```python
from build123d import *

# Parameters (mm, degrees)
BASE_FLANGE1_DEPTH        = 132
HEM2_START                = -107
HEM2_DEPTH                = 96.2
SKETCH31_R                = 12.7
CUT_EXTRUDE1_DEPTH        = 208.181817916
EDGE_FLANGE1_DEPTH        = 96.2
EDGE_FLANGE1_BEND_DEPTH   = 213.4
EDGE_FLANGE1_BEND_2_DEPTH = 96.2
CHAMFER1_SIZE             = 7
SKETCH41_W                = 21.5
SKETCH41_H                = 27.5
CUT_EXTRUDE2_DEPTH        = 208.181817916
LPATTERN1_COUNT           = 3
LPATTERN1_PITCH           = 33.5
SKETCH44_W                = 235
SKETCH44_H                = 10
CUT_EXTRUDE3_DEPTH        = 0.1
EDGE_FLANGE2_DEPTH        = 123.325
EDGE_FLANGE2_START        = 122.925
EDGE_FLANGE2_2_DEPTH      = 0.4
EDGE_FLANGE2_3_DEPTH      = 122.925
EDGE_FLANGE4_START        = -106.9
EDGE_FLANGE4_DEPTH        = 96.1
EDGE_FLANGE4_2_DEPTH      = 96.1
CHAMFER2_SIZE             = 6
SKETCH80_W                = 213.4
SKETCH80_H                = 1
BOSS_EXTRUDE1_DEPTH       = 7
FILLET1_R                 = 1
SKETCH92_W                = 37
SKETCH92_H                = 27.5
CUT_EXTRUDE4_DEPTH        = 208.181817916


# Read off the part's stored shape, not the designer's step: Hem2, Edge-Flange2, Edge-Flange4
# Sheet-metal steps are written as plain solids
with BuildPart() as part:
    # Sketch1 → Base-Flange1 (new body)
    with BuildSketch(Plane(origin=(0, 0, 0), x_dir=(1, 0, 0), z_dir=(0, 1, 0))):
        with BuildLine():
            Line((117.5, 107), (117.5, 10.8))
            ThreePointArc((117.5, 10.8), (114.336753237, 3.163246763), (106.7, 0))
            Line((106.7, 0), (0, 0))
            Line((0, 0), (-106.7, 0))
            ThreePointArc((-106.7, 0), (-114.336753237, 3.163246763), (-117.5, 10.8))
            Line((-117.5, 10.8), (-117.5, 107))
            Line((-117.5, 107), (-116.7, 107))
            Line((-116.7, 107), (-116.7, 10.8))
            ThreePointArc((-116.7, 10.8), (-113.771067812, 3.728932188), (-106.7, 0.8))
            Line((-106.7, 0.8), (0, 0.8))
            Line((0, 0.8), (106.7, 0.8))
            ThreePointArc((106.7, 0.8), (113.771067812, 3.728932188), (116.7, 10.8))
            Line((116.7, 10.8), (116.7, 107))
            Line((116.7, 107), (117.5, 107))
        make_face()
    extrude(amount=BASE_FLANGE1_DEPTH)

    # Hem2 outline → Hem2 (add)
    with BuildSketch(Plane.XY.offset(HEM2_START)):
        with BuildLine():
            Line((-116.45, 123.925), (-115.65, 123.925))
            Line((-115.65, 123.925), (-115.65, 132))
            ThreePointArc((-115.65, 132), (-116.575, 132.925), (-117.5, 132))
            Line((-117.5, 132), (-116.7, 132))
            ThreePointArc((-116.7, 132), (-116.575, 132.125), (-116.45, 132))
            Line((-116.45, 132), (-116.45, 123.925))
        make_face()
        with BuildLine():
            Line((115.65, 123.925), (116.45, 123.925))
            Line((116.45, 123.925), (116.45, 132))
            ThreePointArc((116.45, 132), (116.575, 132.125), (116.7, 132))
            Line((116.7, 132), (117.5, 132))
            ThreePointArc((117.5, 132), (116.575, 132.925), (115.65, 132))
            Line((115.65, 132), (115.65, 123.925))
        make_face()
    extrude(amount=HEM2_DEPTH)

    # Sweep1: sweep along a path in Sketch30
    with BuildLine(Plane(origin=(0, 132, 0), x_dir=(1, 0, 0), z_dir=(0, 1, 0))) as sweep1_path:
        ThreePointArc((-116.7, 10.8), (-113.771067812, 3.728932188), (-106.7, 0.8))
        Line((-106.7, 0.8), (106.7, 0.8))
        ThreePointArc((106.7, 0.8), (113.771067812, 3.728932188), (116.7, 10.8))
    # Sketch29 → Sweep1 (sweep)
    with BuildSketch(Plane.XY.offset(-10.8)):
        with BuildLine():
            Line((-117.5, 132), (-116.7, 132))
            ThreePointArc((-116.7, 132), (-116.575, 132.125), (-116.45, 132))
            Line((-116.45, 132), (-116.45, 123.925))
            Line((-116.45, 123.925), (-115.65, 123.925))
            Line((-115.65, 123.925), (-115.65, 132))
            ThreePointArc((-115.65, 132), (-116.575, 132.925), (-117.5, 132))
        make_face()
    sweep(path=sweep1_path.line)

    # Sketch31 → Cut-Extrude1 (cut, through all)
    with BuildSketch(Plane.XY):
        with Locations((87, 35.2)):
            Circle(SKETCH31_R)
    extrude(amount=-CUT_EXTRUDE1_DEPTH, mode=Mode.SUBTRACT)

    # Edge-Flange1 section (across the edge) → Edge-Flange1 (add)
    with BuildSketch(Plane(origin=(-116.7, -1, -10.8), x_dir=(0, 1, 0), z_dir=(0, 0, -1))):
        with BuildLine():
            Line((-0.8, 1), (-0.8, 7.5))
            Line((-0.8, 7.5), (0, 7.5))
            Line((0, 7.5), (0, 1))
            ThreePointArc((0, 1), (0.292893219, 0.292893219), (1, 0))
            Line((1, 0), (1, -0.8))
            ThreePointArc((1, -0.8), (-0.272792206, -0.272792206), (-0.8, 1))
        make_face()
    extrude(amount=EDGE_FLANGE1_DEPTH)

    # Edge-Flange1 section 2 (across the edge) → Edge-Flange1 bend (add)
    with BuildSketch(Plane(origin=(106.7, -1, -0.8), x_dir=(0, 1, 0), z_dir=(-1, 0, 0))):
        with BuildLine():
            Line((-0.8, 1), (-0.8, 7.5))
            Line((-0.8, 7.5), (0, 7.5))
            Line((0, 7.5), (0, 1))
            ThreePointArc((0, 1), (0.292893219, 0.292893219), (1, 0))
            Line((1, 0), (1, -0.8))
            ThreePointArc((1, -0.8), (-0.272792206, -0.272792206), (-0.8, 1))
        make_face()
    extrude(amount=EDGE_FLANGE1_BEND_DEPTH)

    # Edge-Flange1 section 3 (across the edge) → Edge-Flange1 bend 2 (add)
    with BuildSketch(Plane(origin=(116.7, -1, -107), x_dir=(0, 1, 0), z_dir=(0, 0, 1))):
        with BuildLine():
            Line((-0.8, 1), (-0.8, 7.5))
            Line((-0.8, 7.5), (0, 7.5))
            Line((0, 7.5), (0, 1))
            ThreePointArc((0, 1), (0.292893219, 0.292893219), (1, 0))
            Line((1, 0), (1, -0.8))
            ThreePointArc((1, -0.8), (-0.272792206, -0.272792206), (-0.8, 1))
        make_face()
    extrude(amount=EDGE_FLANGE1_BEND_2_DEPTH)

    # Chamfer1
    chamfer1_edges = [part.edges().sort_by_distance(p)[0] for p in [
        (106.7, -1.4, -8.3),
        (109.2, -1.4, -10.8),
        (-106.7, -1.4, -8.3),
        (-109.2, -1.4, -10.8),
    ]]
    chamfer(chamfer1_edges, length=CHAMFER1_SIZE)

    # Sketch41 → Cut-Extrude2 (cut, through all)
    with BuildSketch(Plane.XY):
        with Locations((-73.45, 102.6)):
            Rectangle(SKETCH41_W, SKETCH41_H)
    cut_extrude2 = extrude(amount=-CUT_EXTRUDE2_DEPTH, mode=Mode.SUBTRACT)

    # LPattern1: Cut-Extrude2 ×3
    with Locations(*[(0, -i * LPATTERN1_PITCH, 0) for i in range(1, LPATTERN1_COUNT)]):
        add(cut_extrude2, mode=Mode.SUBTRACT)

    # Sketch44 → Cut-Extrude3 (cut)
    with BuildSketch(Plane(origin=(0, 0, -107), x_dir=(-1, 0, 0), z_dir=(0, 0, -1))):
        with Locations((0, 127.925)):
            Rectangle(SKETCH44_W, SKETCH44_H)
    extrude(amount=-CUT_EXTRUDE3_DEPTH, mode=Mode.SUBTRACT)

    # Edge-Flange2 outline → Edge-Flange2 (cut)
    with BuildSketch(Plane(origin=(0, 0, 0), x_dir=(1, 0, 0), z_dir=(0, 1, 0))):
        with BuildLine():
            ThreePointArc((116.7, 105.662741699), (117.29411255, 104.6), (117.5, 103.4))
            Line((117.5, 103.4), (117.5, 107))
            Line((117.5, 107), (116.7, 107))
            Line((116.7, 107), (116.7, 105.662741699))
        make_face()
        with BuildLine():
            ThreePointArc((-117.5, 103.4), (-117.29411255, 104.6), (-116.7, 105.662741699))
            Line((-116.7, 105.662741699), (-116.7, 107))
            Line((-116.7, 107), (-117.5, 107))
            Line((-117.5, 107), (-117.5, 103.4))
        make_face()
    extrude(amount=EDGE_FLANGE2_DEPTH, mode=Mode.SUBTRACT)

    # Edge-Flange2 2 outline → Edge-Flange2 2 (cut)
    with BuildSketch(Plane(origin=(0, 0, 0), x_dir=(1, 0, 0), z_dir=(0, 1, 0)).offset(EDGE_FLANGE2_START)):
        with BuildLine():
            ThreePointArc((117.5, 103.4), (117.29411255, 104.6), (116.7, 105.662741699))
            Line((116.7, 105.662741699), (116.7, 103))
            Line((116.7, 103), (117.5, 103))
            Line((117.5, 103), (117.5, 103.4))
        make_face()
        with BuildLine():
            Line((-116.7, 103), (-116.7, 105.662741699))
            ThreePointArc((-116.7, 105.662741699), (-117.29411255, 104.6), (-117.5, 103.4))
            Line((-117.5, 103.4), (-117.5, 103))
            Line((-117.5, 103), (-116.7, 103))
        make_face()
    extrude(amount=EDGE_FLANGE2_2_DEPTH, mode=Mode.SUBTRACT)

    # Edge-Flange2 3 outline → Edge-Flange2 3 (add)
    with BuildSketch(Plane(origin=(0, 0, 0), x_dir=(1, 0, 0), z_dir=(0, 1, 0))):
        with BuildLine():
            Line((113.9, 107), (101.7, 107))
            Line((101.7, 107), (101.7, 106.2))
            Line((101.7, 106.2), (113.9, 106.2))
            ThreePointArc((113.9, 106.2), (115.879898987, 105.379898987), (116.7, 103.4))
            Line((116.7, 103.4), (116.7, 105.662741699))
            ThreePointArc((116.7, 105.662741699), (115.451471863, 106.648528137), (113.9, 107))
        make_face()
        with BuildLine():
            Line((-101.7, 107), (-113.9, 107))
            ThreePointArc((-113.9, 107), (-115.451471863, 106.648528137), (-116.7, 105.662741699))
            Line((-116.7, 105.662741699), (-116.7, 103.4))
            ThreePointArc((-116.7, 103.4), (-115.879898987, 105.379898987), (-113.9, 106.2))
            Line((-113.9, 106.2), (-101.7, 106.2))
            Line((-101.7, 106.2), (-101.7, 107))
        make_face()
    extrude(amount=EDGE_FLANGE2_3_DEPTH)

    # Edge-Flange4 outline → Edge-Flange4 (cut)
    with BuildSketch(Plane.XY.offset(EDGE_FLANGE4_START)):
        with BuildLine():
            ThreePointArc((116.45, 125.725), (116.237450787, 124.876471863), (115.65, 124.228337046))
            Line((115.65, 124.228337046), (115.65, 123.925))
            Line((115.65, 123.925), (116.45, 123.925))
            Line((116.45, 123.925), (116.45, 125.725))
        make_face()
        with BuildLine():
            Line((-115.65, 123.925), (-115.65, 124.228337046))
            ThreePointArc((-115.65, 124.228337046), (-116.237450787, 124.876471863), (-116.45, 125.725))
            Line((-116.45, 125.725), (-116.45, 123.925))
            Line((-116.45, 123.925), (-115.65, 123.925))
        make_face()
    extrude(amount=EDGE_FLANGE4_DEPTH, mode=Mode.SUBTRACT)

    # Edge-Flange4 2 outline → Edge-Flange4 2 (add)
    with BuildSketch(Plane.XY.offset(EDGE_FLANGE4_START)):
        with BuildLine():
            Line((109.45, 123.925), (114.65, 123.925))
            ThreePointArc((114.65, 123.925), (115.172497216, 124.002502784), (115.65, 124.228337046))
            Line((115.65, 124.228337046), (115.65, 125.725))
            ThreePointArc((115.65, 125.725), (115.357106781, 125.017893219), (114.65, 124.725))
            Line((114.65, 124.725), (109.45, 124.725))
            Line((109.45, 124.725), (109.45, 123.925))
        make_face()
        with BuildLine():
            Line((-114.65, 123.925), (-109.45, 123.925))
            Line((-109.45, 123.925), (-109.45, 124.725))
            Line((-109.45, 124.725), (-114.65, 124.725))
            ThreePointArc((-114.65, 124.725), (-115.357106781, 125.017893219), (-115.65, 125.725))
            Line((-115.65, 125.725), (-115.65, 124.228337046))
            ThreePointArc((-115.65, 124.228337046), (-115.172497216, 124.002502784), (-114.65, 123.925))
        make_face()
    extrude(amount=EDGE_FLANGE4_2_DEPTH)

    # Chamfer2
    chamfer2_edges = [part.edges().sort_by_distance(p)[0] for p in [
        (-109.45, 124.325, -10.8),
        (109.45, 124.325, -10.8),
    ]]
    chamfer(chamfer2_edges, length=CHAMFER2_SIZE)

    # Sketch80 → Boss-Extrude1 (add)
    with BuildSketch(Plane(origin=(0, 0, -1.85), x_dir=(-1, 0, 0), z_dir=(0, 0, -1))):
        with Locations((0, 124.425)):
            Rectangle(SKETCH80_W, SKETCH80_H)
    extrude(amount=BOSS_EXTRUDE1_DEPTH)

    # Fillet1
    fillet1_edges = [part.edges().sort_by_distance(p)[0] for p in [
        (0, 124.925, -1.85),
    ]]
    fillet(fillet1_edges, radius=FILLET1_R)

    # Sketch92 → Cut-Extrude4 (cut, through all)
    with BuildSketch(Plane.XY):
        with Locations((-10.7, 102.6)):
            Rectangle(SKETCH92_W, SKETCH92_H)
    extrude(amount=-CUT_EXTRUDE4_DEPTH, mode=Mode.SUBTRACT)


solid = part.part
```
For this review, take the finished solid that the model builds, in its own axes (mm). A direction names the side the tool comes from. Coordinates: 2 decimals unless noted, no trailing zeros. Write each loop counter-clockwise with the first axis right and the second up, starting at its lowest first coordinate (ties: lowest second). Pieces come first, ordered by that corner, then holes. Notation, with made-up numbers: (-3.5, -14.5) - (16.5, -14.5) arc R15 ccw to (16.5, 3.5) - close; hole circle Ø10 at (-28.75, 76). An arc over 180 degrees is marked (long way). Answer in a Markdown table with one row per item. Add a question column.
Q1. We need section D-D, the plane y = 65. State the section outline as (x, z) points, and give its area (3 significant figures).
Q2. We need section A-A, the plane y = 35.2. State the section outline as (x, z) points, and give its area (3 significant figures).
Q3. Tool access review of faces 4 (the flat face through (1, 128, -1.05)), 5 (the cylindrical face through (-113.67, 127.91, -3.98)), 6 (the flat face through (112, 124.725, -60)), 7 (the flat face through (112, -1, -60)): name each direction out of +Z, -Z, +X, -X, +Y, -Y from which nothing blocks a thin tool from reaching the whole face with its end or side.
Q4. For P1, Ø1.6, axis at y = 125, z = -6.5, coming from the -X side; P2, Ø3, axis at x = 112.5, z = -3, coming from the -Y side; P3, Ø2, axis at x = -85, y = 98, coming from the -Z side; P4, Ø23, axis at x = 87, y = 35.2, coming from the -Z side, all flat-tipped, find the tip position at first contact; note any pin that passes through.
Q5. For probe 1 along Y at (x, z) = (88, -6) (3 decimals); probe 2 along X at (y, z) = (12.5, -14); probe 3 along Y at (x, z) = (87, -0.6), list the stretches that pass through material, from the lowest coordinate up.
Q6. Draft analysis for pull direction X (two halves, no side actions). For faces 1 (the flat face through (116, 127, -106.9)), 2 (the flat face through (-103.2, -1.4, -4.8)), 3 (the flat face through (-112.7, -1.4, -14.3)), state which applies: +X half, -X half, draft (parallel to the pull), parting line (faces both ways), or undercut.
Q7. We need section C-C, the plane x = 2. State the section outline as (y, z) points (3 decimals), and give its area (3 significant figures).
Answer list:
| question | item | result |
|---|---|---|
| 1 | outline | (-117.5, -103.4) arc R3.6 ccw to (-113.9, -107) - (-101.7, -107) - (-101.7, -106.2) - (-113.9, -106.2) arc R2.8 cw to (-116.7, -103.4) - (-116.7, -10.8) arc R10 cw to (-106.7, -0.8) - (-84.2, -0.8) - (-84.2, 0) - (-106.7, 0) arc R10.8 ccw to (-117.5, -10.8) - close; (-62.7, -0.8) - (106.7, -0.8) arc R10 cw to (116.7, -10.8) - (116.7, -103.4) arc R2.8 cw to (113.9, -106.2) - (101.7, -106.2) - (101.7, -107) - (113.9, -107) arc R3.6 ccw to (117.5, -103.4) - (117.5, -10.8) arc R10.8 ccw to (106.7, 0) - (-62.7, 0) - close |
| 1 | area | 355 mm2 |
| 2 | outline | (-117.5, -103.4) arc R3.6 ccw to (-113.9, -107) - (-101.7, -107) - (-101.7, -106.2) - (-113.9, -106.2) arc R2.8 cw to (-116.7, -103.4) - (-116.7, -10.8) arc R10 cw to (-106.7, -0.8) - (-84.2, -0.8) - (-84.2, 0) - (-106.7, 0) arc R10.8 ccw to (-117.5, -10.8) - close; (-62.7, -0.8) - (74.3, -0.8) - (74.3, 0) - (-62.7, 0) - close; (99.7, -0.8) - (106.7, -0.8) arc R10 cw to (116.7, -10.8) - (116.7, -103.4) arc R2.8 cw to (113.9, -106.2) - (101.7, -106.2) - (101.7, -107) - (113.9, -107) arc R3.6 ccw to (117.5, -103.4) - (117.5, -10.8) arc R10.8 ccw to (106.7, 0) - (99.7, 0) - close |
| 2 | area | 335 mm2 |
| 3 | face 4 | none |
| 3 | face 5 | -Y |
| 3 | face 6 | -Z, +Y |
| 3 | face 7 | +Z, -Z |
| 4 | P1 | stops at x = -116.92 |
| 4 | P2 | stops at y = 0 |
| 4 | P3 | stops at z = -0.8 |
| 4 | P4 | passes through |
| 5 | probe 1 | y = -1.8 to -1, 123.925 to 124.925 |
| 5 | probe 2 | x = -117.5 to -116.7, 116.7 to 117.5 |
| 5 | probe 3 | y = -1.34 to 22.5, 47.9 to 132.87 |
| 6 | face 1 | draft |
| 6 | face 2 | -X half |
| 6 | face 3 | undercut |
| 7 | outline | (-1.8, -8.3) - (-1, -8.3) - (-1, -1.8) arc R1 cw to (0, -0.8) - (88.85, -0.8) - (88.85, 0) - (0, 0) arc R1.8 ccw to (-1.8, -1.8) - close; (116.35, -0.8) - (132, -0.8) arc R0.125 cw to (132, -1.05) - (123.925, -1.05) - (123.925, -8.85) - (124.925, -8.85) - (124.925, -2.85) arc R1 cw to (125.925, -1.85) - (132, -1.85) arc R0.925 ccw to (132, 0) - (116.35, 0) - close |
| 7 | area | 106 mm2 |
